from build123d import *

# Parameters (mm, degrees)
SKETCH_1_W             = 150
SKETCH_1_H             = 80
SKETCH_1_R             = 1.3
SKETCH_1_R_2           = 22
EXTRUDE_1_DEPTH        = 5
SKETCH_3_R             = 1.55
SKETCH_3_R_2           = 1.582849294
CUT_EXTRUDE_3_DEPTH    = 12.5
CUT_EXTRUDE_5_DEPTH    = 8
FILLET_3_R             = 2
FILLET_3_OF_MIRROR_2_R = 2
EXTRUDE_4_DEPTH        = 5
FILLET_5_R             = 5
SKETCH_11_R            = 1.55
CUT_EXTRUDE_7_DEPTH    = 25
SKETCH_12_R            = 2.05
CUT_EXTRUDE_8_DEPTH    = 10
CUT_EXTRUDE_9_DEPTH    = 10
FILLET_6_R             = 1
SKETCH_14_R            = 2.25
CUT_EXTRUDE_10_DEPTH   = 2.5
EXTRUDE_5_DEPTH        = 5
CHAMFER_1_SIZE         = 20
CHAMFER_1_SIZE2        = 14.360300861
SKETCH_16_R            = 1.55
CUT_EXTRUDE_11_DEPTH   = 10.5


with BuildPart() as part:
    # 草图1 → 凸台-拉伸1 (new body)
    with BuildSketch(Plane.XY):
        with Locations((-5, 0)):
            Rectangle(SKETCH_1_W, SKETCH_1_H)
        with Locations((0, -24.5)):
            Circle(SKETCH_1_R, mode=Mode.SUBTRACT)
        with Locations((-21.217622393, -12.25)):
            Circle(SKETCH_1_R, mode=Mode.SUBTRACT)
        with Locations((-21.217622393, 12.25)):
            Circle(SKETCH_1_R, mode=Mode.SUBTRACT)
        Circle(SKETCH_1_R_2, mode=Mode.SUBTRACT)
        with Locations((0, 24.5)):
            Circle(SKETCH_1_R, mode=Mode.SUBTRACT)
        with Locations((21.217622393, 12.25)):
            Circle(SKETCH_1_R, mode=Mode.SUBTRACT)
        with Locations((21.217622393, -12.25)):
            Circle(SKETCH_1_R, mode=Mode.SUBTRACT)
    extrude(amount=EXTRUDE_1_DEPTH)

    # 草图3 → 切除-拉伸3 (cut)
    with BuildSketch(Plane.XY.offset(5)):
        with Locations((-60, -25)):
            Circle(SKETCH_3_R)
        with Locations((-60, -5)):
            Circle(SKETCH_3_R_2)
        with Locations((-60, 25)):
            Circle(SKETCH_3_R)
        with Locations((-60, 5)):
            Circle(SKETCH_3_R_2)
    extrude(amount=-CUT_EXTRUDE_3_DEPTH, mode=Mode.SUBTRACT)

    # 草图4 → 切除-拉伸5 (cut)
    with BuildSketch(Plane.XY.offset(5)):
        Polygon((-58, 35), (-30, 35), (-58, 11.505210327), align=None)
        Polygon((-35, 25.582872687), (-58, 6.28358117), (-35, 6.28358117), align=None)
    cut_extrude_5 = extrude(amount=-CUT_EXTRUDE_5_DEPTH, mode=Mode.SUBTRACT)

    # 圆角3
    fillet_3_edges = [part.edges().sort_by_distance(p)[0] for p in [
        (-35, 6.28358117, 2.5),
        (-58, 6.28358117, 2.5),
        (-35, 25.582872687, 2.5),
        (-30, 35, 2.5),
        (-58, 11.505210327, 2.5),
        (-58, 35, 2.5),
    ]]
    fillet(fillet_3_edges, radius=FILLET_3_R)

    # 镜向2: 切除-拉伸5 across plane
    add(cut_extrude_5.mirror(Plane.ZX), mode=Mode.SUBTRACT)

    # 圆角3 of 镜向2
    fillet_3_of_mirror_2_edges = [part.edges().sort_by_distance(p)[0] for p in [
        (-35, -6.28358117, 2.5),
        (-58, -6.28358117, 2.5),
        (-35, -25.582872687, 2.5),
        (-30, -35, 2.5),
        (-58, -11.505210327, 2.5),
        (-58, -35, 2.5),
    ]]
    fillet(fillet_3_of_mirror_2_edges, radius=FILLET_3_OF_MIRROR_2_R)

    # 草图10 → 凸台-拉伸4 (add)
    with BuildSketch(Plane.XY.offset(5)):
        Polygon((-80, -40), (-127.053079228, -7.053079228), (-80, 40), align=None)
    extrude(amount=-EXTRUDE_4_DEPTH)

    # 圆角5
    fillet_5_edges = [part.edges().sort_by_distance(p)[0] for p in [
        (-127.053079228, -7.053079228, 2.5),
    ]]
    fillet(fillet_5_edges, radius=FILLET_5_R)

    # 草图11 → 切除-拉伸7 (cut)
    with BuildSketch(Plane.XY.offset(5)):
        with Locations((-15.75, 27.279800219)):
            Circle(SKETCH_11_R)
        with Locations((15.75, 27.279800219)):
            Circle(SKETCH_11_R)
        with Locations((31.5, 0)):
            Circle(SKETCH_11_R)
        with Locations((15.75, -27.279800219)):
            Circle(SKETCH_11_R)
        with Locations((-15.75, -27.279800219)):
            Circle(SKETCH_11_R)
        with Locations((-31.5, 0)):
            Circle(SKETCH_11_R)
    extrude(amount=-CUT_EXTRUDE_7_DEPTH, mode=Mode.SUBTRACT)

    # 草图12 → 切除-拉伸8 (cut)
    with BuildSketch(Plane.XY.offset(5)):
        with Locations((35, 25)):
            Circle(SKETCH_12_R)
        with Locations((65, 25)):
            Circle(SKETCH_12_R)
        with Locations((65, -25)):
            Circle(SKETCH_12_R)
        with Locations((35, -25)):
            Circle(SKETCH_12_R)
    extrude(amount=-CUT_EXTRUDE_8_DEPTH, mode=Mode.SUBTRACT)

    # 草图13 → 切除-拉伸9 (cut)
    with BuildSketch(Plane.XY.offset(5)):
        Polygon((35, 19), (35, -19), (46.4, 0), align=None)
        Polygon((65, -19), (53.6, 0), (65, 19), align=None)
        Polygon((41, 19), (50, 4), (59, 19), align=None)
        Polygon((50, -4), (59, -19), (41, -19), align=None)
    extrude(amount=-CUT_EXTRUDE_9_DEPTH, mode=Mode.SUBTRACT)

    # 圆角6
    fillet_6_edges = [part.edges().sort_by_distance(p)[0] for p in [
        (41, 19, 2.5),
        (59, 19, 2.5),
        (50, 4, 2.5),
        (65, 19, 2.5),
        (65, -19, 2.5),
        (53.6, 0, 2.5),
        (41, -19, 2.5),
        (50, -4, 2.5),
        (59, -19, 2.5),
        (35, 19, 2.5),
        (46.4, 0, 2.5),
        (35, -19, 2.5),
    ]]
    fillet(fillet_6_edges, radius=FILLET_6_R)

    # 草图14 → 切除-拉伸10 (cut)
    with BuildSketch(Plane(origin=(0, 0, 0), x_dir=(-1, 0, 0), z_dir=(0, 0, -1))):
        with Locations((0, 24.5)):
            Circle(SKETCH_14_R)
        with Locations((21.217622393, 12.25)):
            Circle(SKETCH_14_R)
        with Locations((21.217622393, -12.25)):
            Circle(SKETCH_14_R)
        with Locations((0, -24.5)):
            Circle(SKETCH_14_R)
        with Locations((-21.217622393, -12.25)):
            Circle(SKETCH_14_R)
        with Locations((-21.217622393, 12.25)):
            Circle(SKETCH_14_R)
    extrude(amount=-CUT_EXTRUDE_10_DEPTH, mode=Mode.SUBTRACT)

    # 草图15 → 凸台-拉伸5 (add)
    with BuildSketch(Plane(origin=(0, 0, 0), x_dir=(-1, 0, 0), z_dir=(0, 0, -1))):
        Polygon((15.733339697, -85), (80, -40), (-50, -40), (-50, -85), align=None)
        Polygon((-50, -85), (-50, -40), (-180, -40), (-115.733339697, -85), align=None)
    extrude(amount=-EXTRUDE_5_DEPTH)

    # 倒角1
    chamfer_1_edges = [part.edges().sort_by_distance(p)[0] for p in [
        (180, -40, 2.5),
    ]]
    chamfer_1_side = [part.faces().sort_by_distance(p)[0] for p in [
        (147.866669848, -62.5, 2.5),
    ]]
    chamfer(chamfer_1_edges, length=CHAMFER_1_SIZE, length2=CHAMFER_1_SIZE2, reference=chamfer_1_side[0])

    # 草图16 → 切除-拉伸11 (cut)
    with BuildSketch(Plane(origin=(0, 0, 0), x_dir=(-1, 0, 0), z_dir=(0, 0, -1))):
        with Locations((-95, -82)):
            Circle(SKETCH_16_R)
        with Locations((-75, -82)):
            Circle(SKETCH_16_R)
        with Locations((-25, -82)):
            Circle(SKETCH_16_R)
        with Locations((-5, -82)):
            Circle(SKETCH_16_R)
    extrude(amount=-CUT_EXTRUDE_11_DEPTH, mode=Mode.SUBTRACT)


solid = part.part
Model file for the job. Use its own axes, mm. A direction names the side the tool comes from. Round coordinates to 2 decimals unless told otherwise and drop trailing zeros. Loops run counter-clockwise (first coordinate to the right, second up) from the corner with the lowest first, then second, coordinate; pieces in that order, holes last. Notation, with made-up numbers: (-5.5, 15.5) - (49.5, 15.5) arc R15 cw to (49.5, 23.5) - close; hole circle Ø3 at (62, 86). An arc over 180 degrees is marked (long way). Write each question's results on one line, items separated by ' | '.
(1) Saw through at A-A, the plane x = 87. List the corners of the cut face in (y, z).
Answer below:
outline: (-85, 0) - (-40, 0) - (-40, 5) - (-85, 5) - close
(2) 3-axis set-ups, long thin cutter, end or side, ignore diameter. For faces 1 (the flat face through (50, 19, 3)), 2 (the cylindrical face through (-124.28, -6.87, 2.46)): which of +Z, -Z, +X, -X, +Y, -Y reach the whole face in a straight line?
Answer below:
face 1: +Z, -Z | face 2: +Z, -Z, -X
(3) Mould opens along X. For faces 3 (the flat face through (117, -40, 2)), 4 (the flat face through (-102, 18, 3)), 5 (the flat face through (41.41, -8.32, 2.54)), 6 (the flat face through (70, -1, 2)) say: released by +X, released by -X, zero draft, split by the parting line, or undercut.
Answer below:
face 3: zero draft | face 4: released by -X | face 5: undercut | face 6: released by +X
(4) Saw through at C-C, the plane y = -72. List the corners of the cut face in (x, z).
Answer below:
outline: (-34.3, 0) - (134.3, 0) - (134.3, 5) - (-34.3, 5) - close
(5) Wall check: L1, parallel to Y at x = -22.5, z = 1.75; L2, parallel to X at y = -24.5, z = 3.4; L3, parallel to Y at x = -15.5, z = 4.45. Give the ranges that are in metal, low to high.
Answer below:
L1: y = -80.26 to -14.1, -10.4 to 10.4, 14.1 to 40 | L2: x = -102.14 to -61.47, -58.53 to -58, -42.51 to -1.3, 1.3 to 33.01, 36.99 to 63.01, 66.99 to 70 | L3: y = -85 to -28.81, -25.75 to -15.61, 15.61 to 25.75, 28.81 to 40
(6) Saw through at B-B, the plane z = 3.4. Count the separate pieces of the cut face and the enclosed holes in it, then the cut area to 3 significant figures.
Answer below:
separate pieces: 1 | enclosed holes: 33 | area: 19,100 mm^2
(7) Pin check, flat tips, straight feed: pin 1 (3.5 mm diameter, centred on x = -0.5, y = 25, fed in from -Z); pin 2 (10 mm diameter, centred on x = 2, y = 13.5, fed in from -Z); pin 3 (2 mm diameter, centred on x = 20.5, y = -12, fed in from -Z). Stop position of each tip, or through.
Answer below:
pin 1: stops at z = 0 | pin 2: passes through | pin 3: stops at z = 2.5
